For this review, take the finished solid that the model builds, in its own axes (mm). Face numbers are marked on the shaded views. Coordinates: 2 decimals unless noted, no trailing zeros. Loops run counter-clockwise (first coordinate to the right, second up) from the corner with the lowest first, then second, coordinate; pieces in that order, holes last. Notation, with made-up numbers: (-22, 1) -> (37, 1) arc R27 ccw to (37, 21) -> close; hole circle Ø9 at (21.5, 41.25). An arc over 180 degrees is marked (long way). Answer in a Markdown table with one row per item.
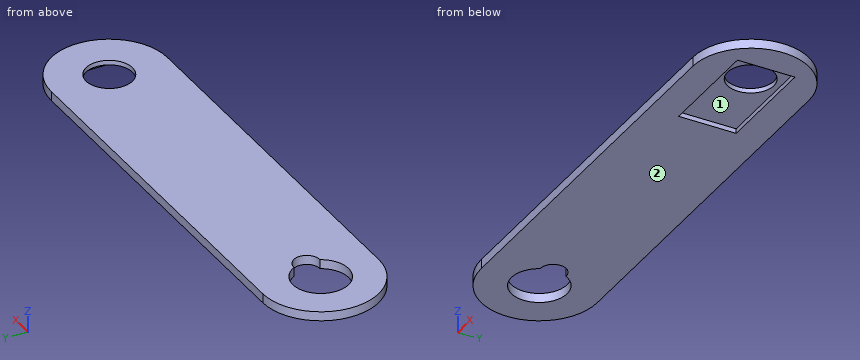
from build123d import *

# Parameters (mm, degrees)
SKETCH1_R           = 0.5
BOSS_EXTRUDE1_DEPTH = 2
CUT_EXTRUDE2_DEPTH  = 2
CUT_EXTRUDE3_DEPTH  = 1
SKETCH5_R           = 5
CUT_EXTRUDE4_DEPTH  = 10


with BuildPart() as part:
    # Sketch1 → Boss-Extrude1 (new body)
    with BuildSketch(Plane.XY):
        with BuildLine():
            Line((32.5, -3.897601476), (-49.5, -3.897601476))
            ThreePointArc((-49.5, -3.897601476), (-62, 8.602398524), (-49.5, 21.102398524))
            Line((-49.5, 21.102398524), (32.5, 21.102398524))
            ThreePointArc((32.5, 21.102398524), (45, 8.602398524), (32.5, -3.897601476))
        make_face()
        with Locations((-49.5, 8.602398524)):
            Circle(SKETCH1_R, mode=Mode.SUBTRACT)
        with Locations((32.5, 8.602398524)):
            Circle(SKETCH1_R, mode=Mode.SUBTRACT)
    extrude(amount=BOSS_EXTRUDE1_DEPTH)

    # Sketch3 → Cut-Extrude2 (cut)
    with BuildSketch(Plane(origin=(0, 0, 0), x_dir=(-1, 0, 0), z_dir=(0, 0, -1))):
        with BuildLine():
            ThreePointArc((44.192592593, 11.400867143), (41.3, 8.602398524), (44.192592593, 5.803929905))
            ThreePointArc((44.192592593, 5.803929905), (55.5, 8.602398524), (44.192592593, 11.400867143))
        make_face()
    extrude(amount=-CUT_EXTRUDE2_DEPTH, mode=Mode.SUBTRACT)

    # Sketch4 → Cut-Extrude3 (cut)
    with BuildSketch(Plane(origin=(0, 0, 0), x_dir=(-1, 0, 0), z_dir=(0, 0, -1))):
        with BuildLine():
            ThreePointArc((-33, 8.602398524), (-32.853553391, 8.955951915), (-32.5, 9.102398524))
            Line((-32.5, 9.102398524), (-32.5, 14.802398524))
            Line((-32.5, 14.802398524), (-38.5, 14.802398524))
            Line((-38.5, 14.802398524), (-38.5, 8.602398524))
            Line((-38.5, 8.602398524), (-33, 8.602398524))
        make_face()
        with BuildLine():
            Line((-32.5, 2.402398524), (-32.5, 8.102398524))
            ThreePointArc((-32.5, 8.102398524), (-32.853553391, 8.248845133), (-33, 8.602398524))
            Line((-33, 8.602398524), (-38.5, 8.602398524))
            Line((-38.5, 8.602398524), (-38.5, 2.402398524))
            Line((-38.5, 2.402398524), (-32.5, 2.402398524))
        make_face()
        with BuildLine():
            Line((-32.5, 14.802398524), (-32.5, 9.102398524))
            ThreePointArc((-32.5, 9.102398524), (-32.146446609, 8.955951915), (-32, 8.602398524))
            Line((-32, 8.602398524), (-15.7, 8.602398524))
            Line((-15.7, 8.602398524), (-15.7, 14.802398524))
            Line((-15.7, 14.802398524), (-32.5, 14.802398524))
        make_face()
        with BuildLine():
            ThreePointArc((-32, 8.602398524), (-32.146446609, 8.248845133), (-32.5, 8.102398524))
            Line((-32.5, 8.102398524), (-32.5, 2.402398524))
            Line((-32.5, 2.402398524), (-15.7, 2.402398524))
            Line((-15.7, 2.402398524), (-15.7, 8.602398524))
            Line((-15.7, 8.602398524), (-32, 8.602398524))
        make_face()
    extrude(amount=-CUT_EXTRUDE3_DEPTH, mode=Mode.SUBTRACT)

    # Sketch5 → Cut-Extrude4 (cut)
    with BuildSketch(Plane.XY.offset(2)):
        with Locations((32.5, 8.602398524)):
            Circle(SKETCH5_R)
    extrude(amount=-CUT_EXTRUDE4_DEPTH, mode=Mode.SUBTRACT)


solid = part.part
Item 1: Take a section at B-B, the plane z = 1.35. State the section outline as (x, y) points.
Worked answers:
| item | result |
|---|---|
| outline | (-49.5, -3.9) -> (32.5, -3.9) arc R12.5 ccw to (32.5, 21.1) -> (-49.5, 21.1) arc R12.5 ccw to start; hole (-44.19, 5.8) arc R2.8 ccw (long way) to (-44.19, 11.4) arc R6 ccw (long way) to start; hole circle Ø10 at (32.5, 8.6) |
Item 2: Take a section at D-D, the plane y = -1.25. State the section outline as (x, z) points, and give its area (3 significant figures).
Worked answers:
| item | result |
|---|---|
| outline | (-57.19, 0) -> (40.19, 0) -> (40.19, 2) -> (-57.19, 2) -> close |
| area | 195 mm² |
Item 3: The part is to be moulded in two halves that separate along Y. For the marked faces 1 and 2, say which applies: +Y half, -Y half, draft (parallel to the pull), parting line (faces both ways), or undercut.
Worked answers:
| item | result |
|---|---|
| face 1 | undercut |
| face 2 | draft |
Item 4: Insertion check: pin 1 (7 mm diameter, centred on x = -49.5, y = 8.6, fed in from +Z); pin 2 (1.1 mm diameter, centred on y = 10.5, z = 0.5, fed in from -X); pin 3 (3.5 mm diameter, centred on x = 25.5, y = 8.5, fed in from -Z). Each pin has a flat end and moves straight along its axis. Give the tip position at first contact, or say it passes through.
Worked answers:
| item | result |
|---|---|
| pin 1 | through |
| pin 2 | x = -61.93 |
| pin 3 | z = 1 |
Item 5: For L1, parallel to X at y = 8.25, z = 1.3; L2, parallel to Y at x = -49.5, z = 1.15; L3, parallel to X at y = 6.25, z = 1.5, list the stretches that pass through material, from the lowest coordinate up.
Worked answers:
| item | result |
|---|---|
| L1 | -62 to -55.49, -41.32 to 27.51, 37.49 to 45 |
| L2 | -3.9 to 2.6, 14.6 to 21.1 |
| L3 | -61.78 to -55.02, -42.58 to 28.09, 36.91 to 44.78 |
Item 6: Take a section at C-C, the plane y = 19.75. State the section outline as (x, z) points.
Worked answers:
| item | result |
|---|---|
| outline | (-55.16, 0) -> (38.16, 0) -> (38.16, 2) -> (-55.16, 2) -> close |
Item 7: Take a section at A-A, the plane x = 24. State the section outline as (y, z) points, and give its area (3 significant figures).
Worked answers:
| item | result |
|---|---|
| outline | (-3.9, 0) -> (2.4, 0) -> (2.4, 1) -> (14.8, 1) -> (14.8, 0) -> (21.1, 0) -> (21.1, 2) -> (-3.9, 2) -> close |
| area | 37.6 mm² |
